```python
from build123d import *

# Parameters (mm, degrees)
SCHIZZO1_W                   = 50
SCHIZZO1_H                   = 12
ESTRUSIONE_ESTRUSIONE1_DEPTH = 3
SCHIZZO2_W                   = 50
SCHIZZO2_H                   = 3
ESTRUSIONE_ESTRUSIONE2_DEPTH = 25
SCHIZZO3_W                   = 66
SCHIZZO3_H                   = 12
ESTRUSIONE_ESTRUSIONE3_DEPTH = 3
SCHIZZO5_R                   = 1.5
TAGLIO_ESTRUSIONE1_DEPTH     = 6
SCHIZZO6_R                   = 1.5
TAGLIO_ESTRUSIONE2_DEPTH     = 6
RACCORDO1_R                  = 1


with BuildPart() as part:
    # Schizzo1 → Estrusione-Estrusione1 (new body)
    with BuildSketch(Plane.XY):
        Rectangle(SCHIZZO1_W, SCHIZZO1_H)
    extrude(amount=ESTRUSIONE_ESTRUSIONE1_DEPTH)

    # Schizzo2 → Estrusione-Estrusione2 (add)
    with BuildSketch(Plane.XY.offset(3)):
        with Locations((0, 4.5)):
            Rectangle(SCHIZZO2_W, SCHIZZO2_H)
    extrude(amount=ESTRUSIONE_ESTRUSIONE2_DEPTH)

    # Schizzo3 → Estrusione-Estrusione3 (add)
    with BuildSketch(Plane.XY.offset(28)):
        Rectangle(SCHIZZO3_W, SCHIZZO3_H)
    extrude(amount=ESTRUSIONE_ESTRUSIONE3_DEPTH)

    # Schizzo5 → Taglio-Estrusione1 (cut)
    with BuildSketch(Plane.XY.offset(31)):
        with Locations((29, 0.28)):
            Circle(SCHIZZO5_R)
        with Locations((-29, 0.28)):
            Circle(SCHIZZO5_R)
    extrude(amount=-TAGLIO_ESTRUSIONE1_DEPTH, mode=Mode.SUBTRACT)

    # Schizzo6 → Taglio-Estrusione2 (cut)
    with BuildSketch(Plane(origin=(0, 0, 0), x_dir=(-1, 0, 0), z_dir=(0, 0, -1))):
        with Locations((-22, -1.5)):
            Circle(SCHIZZO6_R)
        with Locations(Location((22, -1.5, 0), (0, 0, 180))):
            Circle(SCHIZZO6_R)
    extrude(amount=-TAGLIO_ESTRUSIONE2_DEPTH, mode=Mode.SUBTRACT)

    # Raccordo1
    raccordo1_edges = [part.edges().sort_by_distance(p)[0] for p in [
        (-25, -1.5, 3),
        (0, -6, 3),
        (0, 3, 3),
        (-25, 3, 15.5),
        (25, 3, 15.5),
        (-25, 4.5, 28),
        (0, 3, 28),
        (25, 4.5, 28),
        (33, 0, 28),
        (33, -6, 29.5),
        (29, 6, 28),
        (-29, 6, 28),
        (33, 6, 29.5),
        (-33, 0, 28),
        (-33, 6, 29.5),
        (0, -6, 28),
        (-33, -6, 29.5),
        (33, 0, 31),
        (0, 6, 31),
        (-33, 0, 31),
        (0, -6, 31),
        (25, -1.5, 3),
        (0, -6, 0),
        (-25, 0, 0),
        (0, 6, 0),
        (25, 0, 0),
        (25, -6, 1.5),
        (-25, -6, 1.5),
        (-25, 6, 14),
        (25, 6, 14),
    ]]
    fillet(raccordo1_edges, radius=RACCORDO1_R)


solid = part.part
```
Here's how the part is built. I have some questions about the finished solid (model axes, mm). A direction names the side the tool comes from. Round coordinates to 2 decimals unless told otherwise and drop trailing zeros. Order: outer loops, then holes, each group sorted by start corner. A loop starts at its lowest first (then second) coordinate and runs counter-clockwise, first axis right, second up. Notation, with made-up numbers: M 70,37.5 L 100,37.5 A22 ccw 100,76.5 Z; hole C -2.5,71 d7. An arc over 180 degrees is marked long. Answer in a Markdown table with one row per item.
Item 1: I'm going to push flat-ended pins straight in: pin 1 (18.5 mm diameter, centred on x = -3, z = 12, fed in from -Y); pin 2 (3.5 mm diameter, centred on x = -29, y = 0.28, fed in from +Z); pin 3 (1.5 mm diameter, centred on y = 3, z = 5, fed in from -X). Where does each tip first touch, or does it pass through?
A:
| item | result |
|---|---|
| pin 1 | stops at y = -5.66 |
| pin 2 | stops at z = 31 |
| pin 3 | stops at x = -24.97 |
Item 2: Imagine slicing it at C-C, the plane x = 29. Write out the boundary of the cut face in (y, z).
A:
| item | result |
|---|---|
| outline | M -6,29 A1 ccw -5,28 L -1.22,28 L -1.22,31 L -5,31 A1 ccw -6,30 Z; M 1.78,28 L 5,28 A1 ccw 6,29 L 6,30 A1 ccw 5,31 L 1.78,31 Z |
Item 3: Imagine slicing it at B-B, the plane z = 16. Write out the boundary of the cut face in (x, y), and give its area (3 significant figures).
A:
| item | result |
|---|---|
| outline | M -25,4 A1 ccw -24,3 L 24,3 A1 ccw 25,4 L 25,5 A1 ccw 24,6 L -24,6 A1 ccw -25,5 Z |
| area | 149 mm2 |
Item 4: If I drill on L1, parallel to Z at x = -21, y = -4; L2, parallel to Y at x = -29, z = 29.05; L3, parallel to Y at x = 22, z = 1.55, over which ranges is the centre line in solid material (lowest first)? Write a range as from..to.
A:
| item | result |
|---|---|
| L1 | z = 0..3, 28..31 |
| L2 | y = -6..-1.22, 1.78..6 |
| L3 | y = -6..-3, 0..6 |
Item 5: Imagine slicing it at A-A, the plane x = -22. Write out the boundary of the cut face in (y, z), and give its area (3 significant figures).
A:
| item | result |
|---|---|
| outline | M -6,1 A1 ccw -5,0 L -3,0 L -3,3 L -5,3 A1 ccw -6,2 Z; M -6,29 A1 ccw -5,28 L 2,28 A1 cw 3,27 L 3,4 A1 cw 2,3 L 0,3 L 0,0 L 5,0 A1 ccw 6,1 L 6,30 A1 ccw 5,31 L -5,31 A1 ccw -6,30 Z |
| area | 137 mm2 |
Item 6: For faces 4 (the face through (25, 4.4, 11.1)), 5 (the face through (-25, 4.4, 11.1)), 6 (the face through (-23.5, -1.57, 1.48)), 7 (the face through (-30.5, 0.3, 29.5)), 8 (the face through (0, -1, 3)), which set-ups out of +Z, -Z, +X, -X, +Y, -Y let a thin tool reach every point of the face, with its end or its side?
A:
| item | result |
|---|---|
| face 4 | -Z, +X, +Y, -Y |
| face 5 | -Z, -X, +Y, -Y |
| face 6 | -Z |
| face 7 | +Z, -Z |
| face 8 | +X, -X, -Y |
Item 7: Thinking about a two-plate mould opening in Y: for faces 1 (the face through (27.5, 0.3, 29.5)), 2 (the face through (0, -1, 28)), 3 (the face through (0, 3, 15)), which applies, +Y half, -Y half, draft (parallel to the pull), parting line (faces both ways), or undercut?
A:
| item | result |
|---|---|
| face 1 | undercut |
| face 2 | draft |
| face 3 | -Y half |
Item 8: Imagine slicing it at D-D, the plane x = -10. Write out the boundary of the cut face in (y, z), and give its area (3 significant figures).
A:
| item | result |
|---|---|
| outline | M -6,1 A1 ccw -5,0 L 5,0 A1 ccw 6,1 L 6,30 A1 ccw 5,31 L -5,31 A1 ccw -6,30 L -6,29 A1 ccw -5,28 L 2,28 A1 cw 3,27 L 3,4 A1 cw 2,3 L -5,3 A1 ccw -6,2 Z |
| area | 146 mm2 |
